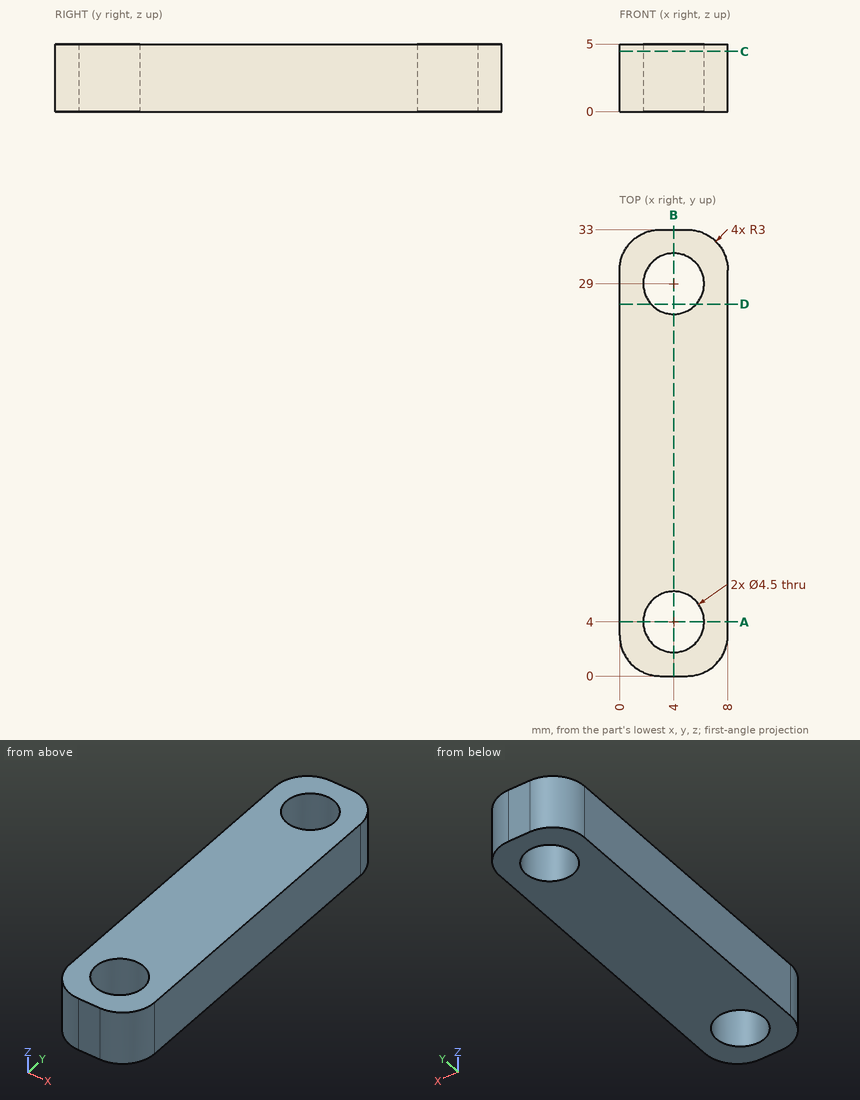
Answer from the drawing. Dimensions are ordinates in mm from the lowest x, y and z of the part. Round coordinates to 2 decimals unless told otherwise and drop trailing zeros. Order: outer loops, then holes, each group sorted by start corner. A loop starts at its lowest first (then second) coordinate and runs counter-clockwise, first axis right, second up. Notation, with made-up numbers: (61.25, 70) - (117.25, 70) arc R23 cw to (117.25, 107) - close; hole circle Ø9 at (60, 56). An arc over 180 degrees is marked (long way). Put each result on its own line as item: value. Start each with the question number.
(1) Find section B-B (x = 4). Give the vertices of the cut face in (y, z).
(2) Straight lines are drawn through the part: probe 1 along Y at (x, z) = (4, 3.35); probe 2 along Y at (x, z) = (4.75, 1.7); probe 3 along X at (y, z) = (31.5, 4.6). For each, find the intervals that lie inside material, in ascending order. Write a range as from..to.
(3) Find section C-C (z = 4.45). Give the vertices of the cut face in (x, y).
(4) Find section A-A (y = 4). Give the vertices of the cut face in (x, z).
(5) Find section D-D (y = 27.5). Give the vertices of the cut face in (x, z), plus the area to 3 significant figures.
Reply:
1. outline: (0, 0) - (1.75, 0) - (1.75, 5) - (0, 5) - close; (6.25, 0) - (26.75, 0) - (26.75, 5) - (6.25, 5) - close; (31.25, 0) - (33, 0) - (33, 5) - (31.25, 5) - close
2. probe 1: 0..1.75, 6.25..26.75, 31.25..33
2. probe 2: 0..1.88, 6.12..26.88, 31.12..33
2. probe 3: 0.4..7.6
3. outline: (0, 3) arc R3 ccw to (3, 0) - (5, 0) arc R3 ccw to (8, 3) - (8, 30) arc R3 ccw to (5, 33) - (3, 33) arc R3 ccw to (0, 30) - close; hole circle Ø4.5 at (4, 4); hole circle Ø4.5 at (4, 29)
4. outline: (0, 0) - (1.75, 0) - (1.75, 5) - (0, 5) - close; (6.25, 0) - (8, 0) - (8, 5) - (6.25, 5) - close
5. outline: (0, 0) - (2.32, 0) - (2.32, 5) - (0, 5) - close; (5.68, 0) - (8, 0) - (8, 5) - (5.68, 5) - close
5. area: 23.2 mm^2
